```python
from build123d import *

# Parameters (mm, degrees)
F0_W     = 18
F0_H     = 17
F1_DEPTH = 10


with BuildPart() as f1:
    # F0 (on Top) → F1 (new body)
    with BuildSketch(Plane.XY):
        with Locations((-55.577677, 38.862)):
            Rectangle(F0_W, F0_H)
        Polygon((-34.21847, 38.862), (-46.577677, 47.362), (-46.577677, 30.362), align=None)
    extrude(amount=F1_DEPTH)


solid = f1.part
```
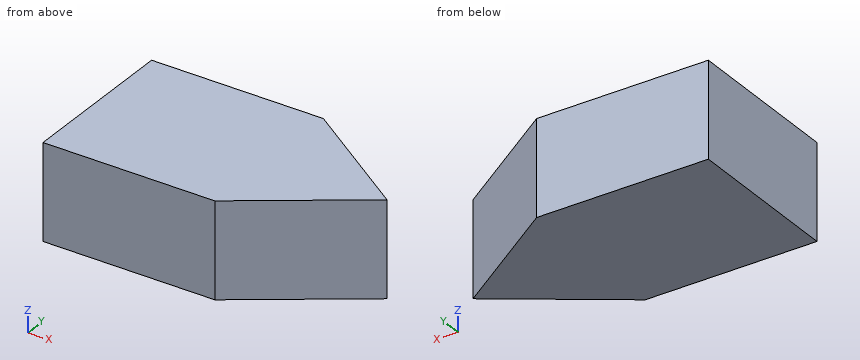
The listing builds one solid part. Answer for the finished solid, in the listing's coordinates (mm). Give positions to 0.01 mm unless a question says otherwise; leave off trailing zeros. Loops run counter-clockwise (first coordinate to the right, second up) from the corner with the lowest first, then second, coordinate; pieces in that order, holes last. Notation, with made-up numbers: (77.25, 26.5) - (119.25, 26.5) arc R33 cw to (119.25, 57.5) - close; hole circle Ø2 at (82, 55.25). An arc over 180 degrees is marked (long way). Answer as CSV lines item,"result". Start each with the question number.
Item 1: A cutting plane is placed at C-C on x = -42. Determine the outline of the cut face in (y, z), then the cut area to 3 significant figures.
Item 2: A cutting plane is placed at A-A on z = 5.5. Determine the outline of the cut face in (x, y).
Item 3: A cutting plane is placed at B-B on y = 42.75. Determine the outline of the cut face in (x, z), then the cut area to 3 significant figures.
Item 4: Each of these flat-tipped pins is pushed along its axis until it touches: pin 1 (2 mm diameter, centred on y = 40.5, z = 6, fed in from +X); pin 2 (5 mm diameter, centred on y = 40.5, z = 2.5, fed in from +X). Where does it stop, or does it pass through?
Item 5: Find the intervals of material crossed by line 1 (X direction, y = 35.5, z = 5.5); line 2 (X direction, y = 34, z = 4); line 3 (Y direction, x = -44, z = 5.25), in increasing order. Write a range as from..to.
Found:
1,outline,"(33.51, 0) - (44.21, 0) - (44.21, 10) - (33.51, 10) - close"
1,area,"107 mm^2"
2,outline,"(-64.58, 30.36) - (-46.58, 30.36) - (-34.22, 38.86) - (-46.58, 47.36) - (-64.58, 47.36) - close"
3,outline,"(-64.58, 0) - (-39.87, 0) - (-39.87, 10) - (-64.58, 10) - close"
3,area,"247 mm^2"
4,pin 1,"stops at x = -35.15"
4,pin 2,"stops at x = -34.22"
5,line 1,"x = -64.58..-39.11"
5,line 2,"x = -64.58..-41.29"
5,line 3,"y = 32.13..45.59"
